Design review of the part built by this model. Coordinates are the model's own, in mm. Face numbers are marked on the shaded views. Coordinates: 2 decimals unless noted, no trailing zeros. Order: outer loops, then holes, each group sorted by start corner. A loop starts at its lowest first (then second) coordinate and runs counter-clockwise, first axis right, second up. Notation, with made-up numbers: (-19.75, 4.5) -> (37.25, 4.5) arc R14 ccw to (37.25, 11.5) -> close; hole circle Ø2 at (46, 37.25). An arc over 180 degrees is marked (long way). Write item = value, one per line.
```python
from build123d import *

# Parameters (mm, degrees)
SKETCH_1_R               = 2.95
EXTRUDE_1_DEPTH          = 9
SKETCH_2_R               = 4.5
SKETCH_2_R_2             = 2.6
EXTRUDE_2_DEPTH          = 0.8
SKETCH_3_R               = 2
CUT_EXTRUDE_1_DEPTH      = 12.022703843
EXTRUDE_3_REACH          = 10.093
PATTERN_CIRCULAR_1_COUNT = 24
CHAMFER_2_SIZE           = 0.5
FILLET_1_R               = 0.2
SKETCH_6_R               = 2.65
SKETCH_6_R_2             = 2
CUT_EXTRUDE_2_DEPTH      = 4
FILLET_2_R               = 0.2


with BuildPart() as part:
    # Эскиз1 → Вытянуть1 (new body)
    with BuildSketch(Plane.XY):
        Circle(SKETCH_1_R)
    extrude(amount=EXTRUDE_1_DEPTH)

    # Эскиз2 → Вытянуть2 (add)
    with BuildSketch(Plane.XY.offset(9)):
        Circle(SKETCH_2_R)
        Circle(SKETCH_2_R_2, mode=Mode.SUBTRACT)
    extrude(amount=-EXTRUDE_2_DEPTH)

    # Эскиз3 → Вырез-Вытянуть1 (cut, through all)
    with BuildSketch(Plane.XY.offset(9)):
        Circle(SKETCH_3_R)
    extrude(amount=-CUT_EXTRUDE_1_DEPTH, mode=Mode.SUBTRACT)

    # Эскиз4 → Вытянуть3 (add, up to next)
    with BuildSketch(Plane.XY.offset(5), mode=Mode.PRIVATE) as extrude_3_sk1:
        with BuildLine():
            Line((0.15, 2.946183973), (-0.15, 2.946183973))
            ThreePointArc((-0.15, 2.946183973), (0, 3.096183973), (0.15, 2.946183973))
        make_face()
    extrude_3_tool1 = extrude(extrude_3_sk1.sketch, amount=EXTRUDE_3_REACH, mode=Mode.PRIVATE) - part.part
    extrude_3 = extrude_3_tool1.solids().sort_by_distance((0, 3.009846, 5))[0]
    add(extrude_3)

    # Круговой массив1: Вытянуть3 ×24 about axis
    pattern_circular_1_axis = Axis((0, 0, 0), (0, 0, 1))
    for i in range(1, PATTERN_CIRCULAR_1_COUNT):
        add(extrude_3.rotate(pattern_circular_1_axis, i * 360 / PATTERN_CIRCULAR_1_COUNT))

    # Фаска2
    chamfer_2_edges = [part.edges().sort_by_distance(p)[0] for p in [
        (-2.95, 0, 0),
    ]]
    chamfer(chamfer_2_edges, length=CHAMFER_2_SIZE)

    # Скругление1
    fillet_1_edges = [part.edges().sort_by_distance(p)[0] for p in [
        (-4.5, 0, 9),
        (-4.5, 0, 8.2),
    ]]
    fillet(fillet_1_edges, radius=FILLET_1_R)

    # Эскиз6 → Вырез-Вытянуть2 (cut)
    with BuildSketch(Plane.XY.offset(9)):
        Circle(SKETCH_6_R)
        Circle(SKETCH_6_R_2, mode=Mode.SUBTRACT)
    extrude(amount=-CUT_EXTRUDE_2_DEPTH, mode=Mode.SUBTRACT)

    # Скругление2
    fillet_2_edges = [part.edges().sort_by_distance(p)[0] for p in [
        (-2.65, 0, 9),
    ]]
    fillet(fillet_2_edges, radius=FILLET_2_R)


solid = part.part
```
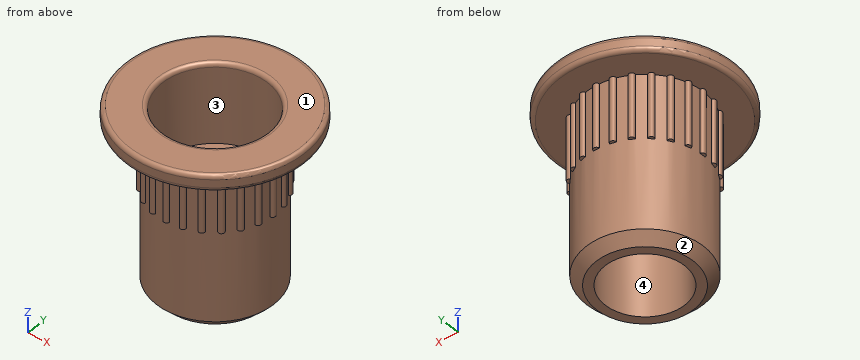
(1) Insertion check: pin 1 (3 mm diameter, centred on x = 2.5, z = 7, fed in from -Y); pin 2 (3.5 mm diameter, centred on x = 0, y = 0, fed in from -Z); pin 3 (2 mm diameter, centred on y = 0.5, z = 3, fed in from +X); pin 4 (2 mm diameter, centred on x = 1.5, z = 1, fed in from +Y). Each pin has a flat end and moves straight along its axis. Give the tip position at first contact, or say it passes through.
Report:
pin_1 = -4.12
pin_2 = through
pin_3 = 2.95
pin_4 = 2.91
(2) We need section A-A (y = 0). Write out the cut boundary in (x, z).
Report:
outline = (-4.5, 8.4) arc R0.2 ccw to (-4.3, 8.2) -> (-3.1, 8.2) -> (-3.1, 5) -> (-2.95, 5) -> (-2.95, 0.5) -> (-2.45, 0) -> (-2, 0) -> (-2, 5) -> (-2.65, 5) -> (-2.65, 8.8) arc R0.2 ccw to (-2.85, 9) -> (-4.3, 9) arc R0.2 ccw to (-4.5, 8.8) -> close; (2, 0) -> (2.45, 0) -> (2.95, 0.5) -> (2.95, 5) -> (3.1, 5) -> (3.1, 8.2) -> (4.3, 8.2) arc R0.2 ccw to (4.5, 8.4) -> (4.5, 8.8) arc R0.2 ccw to (4.3, 9) -> (2.85, 9) arc R0.2 ccw to (2.65, 8.8) -> (2.65, 5) -> (2, 5) -> close
(3) The part is to be moulded in two halves that separate along X. For the marked faces 1, 2, 3 and 4, say which applies: released by +X, released by -X, zero draft, split by the parting line, or undercut.
Report:
face_1 = zero draft
face_2 = split by the parting line
face_3 = undercut
face_4 = undercut
(4) For L1, parallel to Y at x = 0, z = 1.9; L2, parallel to Y at x = 0, z = 7.8; L3, parallel to Z at x = 0, y = 4, list the stretches that pass through material, from the lowest coordinate up.
Report:
L1 = -2.95 to -2, 2 to 2.95
L2 = -3.1 to -2.65, 2.65 to 3.1
L3 = 8.2 to 9
(5) We need section C-C (z = 4). Write out the cut boundary in (x, y).
Report:
outline = circle Ø5.9 at (0, 0); hole circle Ø4 at (0, 0)
